Here's how the part is built. I have some questions about the finished solid (model axes, mm). A direction names the side the tool comes from. Round coordinates to 2 decimals unless told otherwise and drop trailing zeros. Loops run counter-clockwise (first coordinate to the right, second up) from the corner with the lowest first, then second, coordinate; pieces in that order, holes last. Notation, with made-up numbers: M 81,74.5 L 95,74.5 A31 ccw 95,99.5 Z; hole C 84,30 d10. An arc over 180 degrees is marked long. Use a Markdown table: item, result.
from build123d import *

# Parameters (mm, degrees)
F1_DEPTH       = 2
F3_DEPTH       = 15
F5_D           = 3.5
F5_CBORE_D     = 10
F5_CBORE_DEPTH = 14
F7_D           = 3.5


with BuildPart() as f1:
    # F0 (on Top) → F1 (new body)
    with BuildSketch(Plane.XY):
        Polygon((7.5, -7.5), (-7.5, 7.5), (-7.5, -7.5), align=None)
        Polygon((7.5, 7.5), (-7.5, 7.5), (7.5, -7.5), align=None)
    extrude(amount=F1_DEPTH)

    # F2 (on face) → F3 (join)
    with BuildSketch(Plane.XY.offset(2)):
        Polygon((6.5, -6.5), (-6.5, 6.5), (-6.5, -6.5), align=None)
        Polygon((6.5, 6.5), (-6.5, 6.5), (6.5, -6.5), align=None)
    extrude(amount=F3_DEPTH)

    # F5 (through all)
    with Locations(Plane.XY.offset(17)):
        with Locations((0, 0)):
            CounterBoreHole(F5_D / 2, F5_CBORE_D / 2, F5_CBORE_DEPTH)

    # F7 (through all)
    with Locations(Plane.XZ.offset(6.5)):
        with Locations((0, 9.5)):
            Hole(F7_D / 2)


solid = f1.part
1. Which directions (+Z, -Z, +X, -X, +Y, -Y) give clear straight access to the entire face, cutting with the end or side of a thin tool? Please do faces 5 (the face through (-7.5, 0, 1)), 6 (the face through (-6.5, 0, 9)), 7 (the face through (2, 6.5, 8)), 8 (the face through (-2, -6.5, 8)), 9 (the face through (4.619, -1.915, 10.098)).
Answer sheet:
| item | result |
|---|---|
| face 5 | +Z, -Z, -X, +Y, -Y |
| face 6 | +Z, -X, +Y, -Y |
| face 7 | +Z, +X, -X, +Y |
| face 8 | +Z, +X, -X, -Y |
| face 9 | +Z |
2. Imagine slicing it at A-A, the plane y = 0. Write out the boundary of the cut face in (x, z).
Answer sheet:
| item | result |
|---|---|
| outline | M -7.5,0 L -1.75,0 L -1.75,3 L -5,3 L -5,17 L -6.5,17 L -6.5,2 L -7.5,2 Z; M 1.75,0 L 7.5,0 L 7.5,2 L 6.5,2 L 6.5,17 L 5,17 L 5,3 L 1.75,3 Z |
3. Imagine slicing it at C-C, the plane x = 0. Write out the boundary of the cut face in (y, z), then the cut area to 3 significant figures.
Answer sheet:
| item | result |
|---|---|
| outline | M -7.5,0 L -1.75,0 L -1.75,3 L -5,3 L -5,7.75 L -6.5,7.75 L -6.5,2 L -7.5,2 Z; M -6.5,11.25 L -5,11.25 L -5,17 L -6.5,17 Z; M 1.75,0 L 7.5,0 L 7.5,2 L 6.5,2 L 6.5,7.75 L 5,7.75 L 5,3 L 1.75,3 Z; M 5,11.25 L 6.5,11.25 L 6.5,17 L 5,17 Z |
| area | 64.0 mm2 |
4. Imagine slicing it at B-B, the plane z = 9.5. Write out the boundary of the cut face in (x, y).
Answer sheet:
| item | result |
|---|---|
| outline | M -6.5,-6.5 L -1.75,-6.5 L -1.75,-4.68 A5 cw -1.75,4.68 L -1.75,6.5 L -6.5,6.5 Z; M 1.75,-6.5 L 6.5,-6.5 L 6.5,6.5 L 1.75,6.5 L 1.75,4.68 A5 cw 1.75,-4.68 Z |
5. Imagine slicing it at D-D, the plane y = -6.25. Write out the boundary of the cut face in (x, z), then the cut area to 3 significant figures.
Answer sheet:
| item | result |
|---|---|
| outline | M -7.5,0 L 7.5,0 L 7.5,2 L 6.5,2 L 6.5,17 L -6.5,17 L -6.5,2 L -7.5,2 Z; hole C 0,9.5 d3.5 |
| area | 215 mm2 |
6. For pin 1 Ø6.5 at (x, z) = (2.5, 8.5) entering from +Y; pin 2 Ø6.5 at (y, z) = (1.5, 6) entering from -X; pin 3 Ø5.5 at (x, z) = (0, 9.5) entering from -Y, each with a flat end and sliding along its axis, tell me the tip position at first contact or that it passes through.
Answer sheet:
| item | result |
|---|---|
| pin 1 | y = 6.5 |
| pin 2 | x = -6.5 |
| pin 3 | y = -6.5 |
7. We'd pull the mould along Z, two halves only. Please class faces 1 (the face through (-1.669, 5.605, 10.026)), 2 (the face through (6.5, 0, 9)), 3 (the face through (-2, 0, 0)), 4 (the face through (-1.669, -5.579, 10.026)): +Z half, -Z half, draft (parallel to the pull), parting line (faces both ways), or undercut.
Answer sheet:
| item | result |
|---|---|
| face 1 | undercut |
| face 2 | draft |
| face 3 | -Z half |
| face 4 | undercut |
8. I need wall thicknesses on probe 1 along Y at (x, z) = (0, 1); probe 2 along Y at (x, z) = (6, 6); probe 3 along X at (y, z) = (-5.65, 9.5). Which ranges of each line are inside material? Lowest first, please. Write a range as from..to.
Answer sheet:
| item | result |
|---|---|
| probe 1 | -7.5..-1.75, 1.75..7.5 |
| probe 2 | -6.5..6.5 |
| probe 3 | -6.5..-1.75, 1.75..6.5 |
